Autodesk Inventor part; units mm, degrees
ref_plane "YZ Plane" through (0, 0, 0) normal (1, 0, 0) x (0, 1, 0)
ref_plane "XZ Plane" through (0, 0, 0) normal (0, 1, 0) x (-1, 0, 0)
ref_plane "XY Plane" through (0, 0, 0) normal (0, 0, 1) x (1, 0, 0)
sketch "Sketch1" plane through (0, 0, 0) normal (0, 0, 1) x (1, 0, 0)
  line L0 (0, 0) -> (150, 0)
  line L1 (150, 0) -> (150, 80)
  line L2 (150, 80) -> (0, 80)
  line L3 (0, 80) -> (0, 0)
  dimension "d0" = 150
  dimension "d1" = 80
extrude "Extrusion1" add sketch "Sketch1" along normal blind 3
sketch "Sketch2" plane through (0, 0, 3) normal (0, 0, 1) x (1, 0, 0)
  line L0 (0, 80) -> (0, 0)
  line L1 (150, 0) -> (150, 80)
  line L2 (3, 80) -> (3, 53.3333)
  line L3 (3, 53.3333) -> (0, 53.3333)
  line L4 (0, 53.3333) -> (0, 26.6667)
  line L5 (0, 26.6667) -> (3, 26.6667)
  line L6 (3, 26.6667) -> (3, 0)
  line L7 (0, 80) -> (0, 53.3333)
  line L8 (0, 26.6667) -> (0, 0)
  line L9 (147, 80) -> (147, 53.3333)
  line L10 (147, 53.3333) -> (150, 53.3333)
  line L11 (150, 53.3333) -> (150, 26.6667)
  line L12 (150, 26.6667) -> (147, 26.6667)
  line L13 (147, 26.6667) -> (147, 0)
  line L14 (150, 0) -> (150, 26.6667)
  line L15 (150, 53.3333) -> (150, 80)
  line L16 (0, 26.6667) -> (0, 0)
  line L17 (0, 0) -> (0, 3)
  line L18 (0, 3) -> (30, 3)
  line L19 (30, 3) -> (30, 0)
  line L20 (30, 0) -> (60, 0)
  line L21 (0, 0) -> (150, 0)
  line L22 (60, 0) -> (60, 3)
  line L23 (60, 3) -> (90, 3)
  line L24 (90, 3) -> (90, 0)
  line L25 (90, 0) -> (120, 0)
  line L26 (120, 0) -> (120, 3)
  line L27 (120, 3) -> (150, 3)
  line L28 (0, 80) -> (0, 77)
  line L29 (0, 77) -> (30, 77)
  line L30 (30, 77) -> (30, 80)
  line L31 (60, 80) -> (60, 77)
  line L32 (30, 80) -> (60, 80)
  line L33 (0, 80) -> (150, 80)
  line L34 (60, 77) -> (90, 77)
  line L35 (90, 77) -> (90, 80)
  line L36 (120, 80) -> (120, 77)
  line L37 (120, 77) -> (150, 77)
  line L38 (90, 80) -> (120, 80)
  line L39 (0, 0) -> (30, 0)
  line L40 (0, 0) -> (150, 0)
  line L41 (120, 0) -> (150, 0)
  line L42 (150, 0) -> (150, 80)
  line L43 (150, 80) -> (120, 80)
  line L44 (150, 80) -> (0, 80)
  line L45 (30, 80) -> (0, 80)
  dimension "d4" = 3
  dimension "d5" = 26.6667
  dimension "d6" = 26.6667
  dimension "d7" = 3
  dimension "d8" = 26.6667
  dimension "d9" = 26.6667
  dimension "d10" = 3
  dimension "d11" = 30
  dimension "d12" = 30
  dimension "d13" = 30
  dimension "d14" = 30
extrude "Extrusion2" cut sketch "Sketch2" against normal blind 3 contours L33 L2 L29 L0 | L29 L2 L3 L0 | L33 L30 L29 L2 | L5 L6 L18 L0 | L33 L35 L34 L31 | L18 L6 L21 L0 | L18 L19 L21 L6 | L33 L9 L37 L36 | L33 L1 L37 L9 | L37 L1 L10 L9 | L22 L23 L24 L21 | L26 L27 L13 L21 | L1 L27 L13 L12 | L13 L27 L1 L21
sketch "Sketch3" plane through (0, 0, 3) normal (0, 0, 1) x (1, 0, 0)
  line L0 (60, 77) -> (90, 77)
  line L1 (90, 3) -> (60, 3)
  line L2 (0, 53.3333) -> (0, 26.6667)
  line L3 (150, 26.6667) -> (150, 53.3333)
  line L4 (80, 40) -> (80, 35)
  line L5 (80, 35) -> (75, 35)
  line L6 (75, 35) -> (75, 40)
  line L7 (75, 40) -> (80, 40)
  circle A0 centre (32.0086, 37.5) radius 2.5
  circle A1 centre (120.9557, 37.5) radius 2.5
  point P0 (0, 0)
  dimension "d22" = 5
  dimension "d23" = 5
  dimension "d24" = 5
  dimension "d25" = 5
extrude "Extrusion3" cut sketch "Sketch3" against normal blind 3
properties part number "TAPA4"
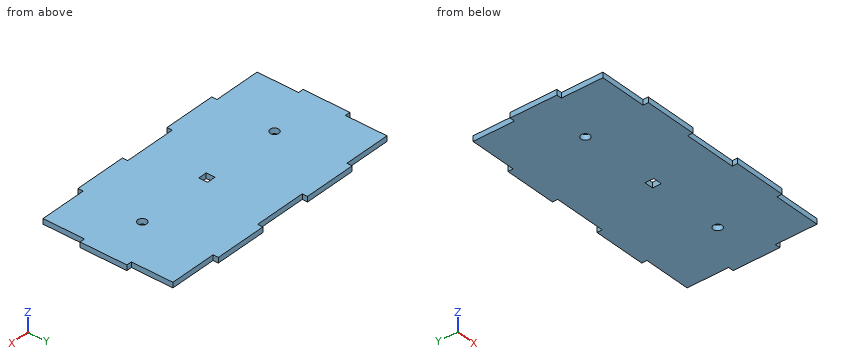
The model under review builds one solid part; all positions refer to its coordinate system, in mm. Give positions to 0.01 mm unless a question says otherwise; leave off trailing zeros. Order: outer loops, then holes, each group sorted by start corner. A loop starts at its lowest first (then second) coordinate and runs counter-clockwise, first axis right, second up. Notation, with made-up numbers: (81, -8.75) - (124, -8.75) arc R20 cw to (124, 4.25) - close; hole circle Ø4 at (67.5, 77.5). An arc over 180 degrees is marked (long way). Use CSV: the item, a comma, the result in double quotes. Start each with the question number.
Q1. We need section A-A, the plane z = 1.7. State how many separate pieces and enclosed holes the cut face has, and give its area (3 significant figures).
Q2. To check wall thickness, follow line 1 along Y through (x, z) = (69, 2.85); line 2 along X through (y, z) = (59.5, 2.6); line 3 along Y through (x, z) = (33, 2.5). State the ranges of each line that lie inside material, in increasing order. Write a range as [from, to].
Q3. We need section B-B, the plane y = 37.5. Write out the cut boundary in (x, z), and give its area (3 significant figures).
Q4. We need section D-D, the plane y = 68.5. Write out the cut boundary in (x, z).
Q5. We need section C-C, the plane x = 17.5. Write out the cut boundary in (y, z), and give its area (3 significant figures).
Q6. Clearance check with flat-ended pins moving along their axes: pin 1 Ø0.9 at (y, z) = (63.5, 1.5) entering from -X; pin 2 Ø1.5 at (y, z) = (13.5, 2) entering from +X; pin 3 Ø0.9 at (x, z) = (68.5, 1) entering from +Y; pin 4 Ø5 at (x, y) = (72.5, 57.5) entering from -Z. State where each tip first meets the part, or that it passes through.
Outcome:
1,separate pieces,"1"
1,enclosed holes,"3"
1,area,"11,100 mm^2"
2,line 1,"y = [3, 77]"
2,line 2,"x = [3, 147]"
2,line 3,"y = [0, 35.2], [39.8, 80]"
3,outline,"(0, 0) - (29.51, 0) - (29.51, 3) - (0, 3) - close; (34.51, 0) - (75, 0) - (75, 3) - (34.51, 3) - close; (80, 0) - (118.46, 0) - (118.46, 3) - (80, 3) - close; (123.46, 0) - (150, 0) - (150, 3) - (123.46, 3) - close"
3,area,"405 mm^2"
4,outline,"(3, 0) - (147, 0) - (147, 3) - (3, 3) - close"
5,outline,"(3, 0) - (77, 0) - (77, 3) - (3, 3) - close"
5,area,"222 mm^2"
6,pin 1,"stops at x = 3"
6,pin 2,"stops at x = 147"
6,pin 3,"stops at y = 77"
6,pin 4,"stops at z = 0"
